CAD build for the part. Positions are in the model's coordinates, mm. A direction names the side the tool comes from. Round coordinates to 2 decimals unless told otherwise and drop trailing zeros. Order: outer loops, then holes, each group sorted by start corner. A loop starts at its lowest first (then second) coordinate and runs counter-clockwise, first axis right, second up. Notation, with made-up numbers: (64.5, 11.5) - (70.5, 11.5) arc R20 ccw to (70.5, 50.5) - close; hole circle Ø5 at (84, -32.5). An arc over 180 degrees is marked (long way). Write item = value, one per line.
from build123d import *

# Parameters (mm, degrees)
F1_DEPTH = 57.15
F2_R     = 9.94537
F3_DEPTH = 88.9
F5_DEPTH = 88.9
F6_W     = 76.2
F6_H     = 44.45
F7_DEPTH = 7.9375
F8_R     = 10.3251
F9_DEPTH = 25.4
F10_R    = 6.35


with BuildPart() as f1:
    # F0 (on Right) → F1 (new body)
    with BuildSketch(Plane.YZ):
        with BuildLine():
            ThreePointArc((0, 12.7), (3.7197438789, 3.7197438789), (12.7, 0))
            Line((12.7, 0), (76.2, 0))
            ThreePointArc((76.2, 0), (85.1802561211, 3.7197438789), (88.9, 12.7))
            Line((88.9, 12.7), (88.9, 73.025))
            Line((88.9, 73.025), (80.9625, 73.025))
            Line((80.9625, 73.025), (80.9625, 12.7))
            ThreePointArc((80.9625, 12.7), (79.5675960454, 9.3324039546), (76.2, 7.9375))
            Line((76.2, 7.9375), (12.7, 7.9375))
            ThreePointArc((12.7, 7.9375), (9.3324039546, 9.3324039546), (7.9375, 12.7))
            Line((7.9375, 12.7), (7.9375, 73.025))
            Line((7.9375, 73.025), (0, 73.025))
            Line((0, 73.025), (0, 12.7))
        make_face()
    extrude(amount=F1_DEPTH)

    # F2 (on face) → F3 (cut)
    with BuildSketch(Plane.XZ):
        with Locations((28.575, 44.45)):
            Circle(F2_R)
    extrude(amount=-F3_DEPTH, mode=Mode.SUBTRACT)

    # F4 (on face) → F5 (cut)
    with BuildSketch(Plane.XZ):
        with BuildLine():
            ThreePointArc((0, 44.45), (8.3694237276, 64.6555762724), (28.575, 73.025))
            Line((28.575, 73.025), (0, 73.025))
            Line((0, 73.025), (0, 44.45))
        make_face()
        with BuildLine():
            ThreePointArc((28.575, 73.025), (48.7805762724, 64.6555762724), (57.15, 44.45))
            Line((57.15, 44.45), (57.15, 73.025))
            Line((57.15, 73.025), (28.575, 73.025))
        make_face()
    extrude(amount=-F5_DEPTH, mode=Mode.SUBTRACT)

    # F6 (on face) → F7 (join)
    with BuildSketch(Plane.XY.offset(7.9375)):
        with Locations((95.25, 44.45)):
            Rectangle(F6_W, F6_H)
    extrude(amount=-F7_DEPTH)

    # F8 (on face) → F9 (cut)
    with BuildSketch(Plane.XY.offset(7.9375)):
        with Locations((73.025, 44.45)):
            Circle(F8_R)
        with Locations((111.125, 44.45)):
            Circle(F8_R)
        with BuildLine():
            ThreePointArc((111.125, 66.675), (126.8404482119, 60.1654482119), (133.35, 44.45))
            Line((133.35, 44.45), (133.35, 66.675))
            Line((133.35, 66.675), (111.125, 66.675))
        make_face()
        with BuildLine():
            Line((133.35, 22.225), (133.35, 44.45))
            ThreePointArc((133.35, 44.45), (126.8404482119, 28.7345517881), (111.125, 22.225))
            Line((111.125, 22.225), (133.35, 22.225))
        make_face()
    extrude(amount=-F9_DEPTH, mode=Mode.SUBTRACT)

    # F10
    f10_edges = [f1.edges().sort_by_distance(p)[0] for p in [
        (57.15, 22.225, 3.96875),
        (57.15, 66.675, 3.96875),
    ]]
    fillet(f10_edges, radius=F10_R)


solid = f1.part
(1) Pull direction X, two halves, no side cores. Call faces 1 (the cylindrical face through (120.973, 47.551, 4.024)), 2 (the flat face through (57.15, 83, 23)), 3 (the flat face through (87, 66.675, 4)): released by +X, released by -X, zero draft, split by the parting line, or undercut.
Solved:
face_1 = undercut
face_2 = released by +X
face_3 = zero draft
(2) Tool access for faces 4 (the flat face through (87, 22.225, 4)), 5 (the cylindrical face through (28.175, 9.37, 9.296)), 6 (the flat face through (22, 88.9, 36)): list every direction of +Z, -Z, +X, -X, +Y, -Y with a clear straight run to the whole face (end or side of a thin tool).
Solved:
face_4 = +Z, -Z, +X, -Y
face_5 = +Z, +X, -X
face_6 = +Z, -Z, +X, -X, +Y
(3) Drop flat-ended pins along their axis: pin 1 (12 mm diameter, centred on x = 28.575, z = 44.45, fed in from +Y); pin 2 (2 mm diameter, centred on x = 33.5, y = 11, fed in from -Z); pin 3 (8.5 mm diameter, centred on x = 90.5, z = 3.5, fed in from +Y) (3 decimals); pin 4 (1.5 mm diameter, centred on x = 68.5, y = 35.5, fed in from +Z). Give the stop position or say it passes through.
Solved:
pin_1 = through
pin_2 = 0.02
pin_3 = 66.675
pin_4 = 7.94
(4) Band-saw the part on B-B on x = 25. List the corners of the cut face in (y, z) (1 decimal), plus the area to 3 significant figures.
Solved:
outline = (0, 12.7) arc R12.7 ccw to (12.7, 0) - (76.2, 0) arc R12.7 ccw to (88.9, 12.7) - (88.9, 35.2) - (81, 35.2) - (81, 12.7) arc R4.8 cw to (76.2, 7.9) - (12.7, 7.9) arc R4.8 cw to (7.9, 12.7) - (7.9, 35.2) - (0, 35.2) - close; (0, 53.7) - (7.9, 53.7) - (7.9, 72.8) - (0, 72.8) - close; (81, 53.7) - (88.9, 53.7) - (88.9, 72.8) - (81, 72.8) - close
area = 1,380 mm²
(5) Band-saw the part on A-A on z = 60. List the corners of the cut face in (x, y).
Solved:
outline = (4.6, 0) - (52.55, 0) - (52.55, 7.94) - (4.6, 7.94) - close; (4.6, 80.96) - (52.55, 80.96) - (52.55, 88.9) - (4.6, 88.9) - close
(6) Band-saw the part on D-D on y = 28.5. List the corners of the cut face in (x, z).
Solved:
outline = (0, 0) - (126.6, 0) - (126.6, 7.94) - (0, 7.94) - close
(7) Probe line 1 along Y through (x, z) = (47, 54.5); line 2 along X through (y, z) = (6, 44); line 3 along X through (y, z) = (83, 9). List the from-to ranges inside material, lowest first.
Solved:
line_1 = 0 to 7.94, 80.96 to 88.9
line_2 = 0 to 18.64, 38.51 to 57.15
line_3 = 0 to 57.15
(8) Band-saw the part on C-C on x = 69. List the corners of the cut face in (y, z) (1 decimal), plus the area to 3 significant figures.
Solved:
outline = (22.2, 0) - (34.9, 0) - (34.9, 7.9) - (22.2, 7.9) - close; (54, 0) - (66.7, 0) - (66.7, 7.9) - (54, 7.9) - close
area = 202 mm²
